from build123d import *

# Parameters (mm, degrees)
SKETCH1_R          = 8
EXTRUDE1_DEPTH     = 1102
SKETCH3_R          = 8
SKETCH3_R_2        = 6
CUT_EXTRUDE1_DEPTH = 54
SKETCH4_R          = 8
SKETCH4_R_2        = 6
CUT_EXTRUDE2_DEPTH = 20
SKETCH5_R          = 6
EXTRUDE2_DEPTH     = 4.4
SKETCH6_R          = 8
SKETCH6_R_2        = 6
EXTRUDE3_DEPTH     = 3
SKETCH7_R          = 8
SKETCH7_R_2        = 6
EXTRUDE4_DEPTH     = 3


with BuildPart() as part:
    # Sketch1 → Extrude1 (new body)
    with BuildSketch(Plane.XY):
        Circle(SKETCH1_R)
    extrude(amount=EXTRUDE1_DEPTH)

    # Sketch3 → Cut-Extrude1 (cut)
    with BuildSketch(Plane.XY.offset(1102)):
        Circle(SKETCH3_R)
        Circle(SKETCH3_R_2, mode=Mode.SUBTRACT)
    extrude(amount=-CUT_EXTRUDE1_DEPTH, mode=Mode.SUBTRACT)

    # Sketch4 → Cut-Extrude2 (cut)
    with BuildSketch(Plane(origin=(0, 0, 0), x_dir=(-1, 0, 0), z_dir=(0, 0, -1))):
        Circle(SKETCH4_R)
        Circle(SKETCH4_R_2, mode=Mode.SUBTRACT)
    extrude(amount=-CUT_EXTRUDE2_DEPTH, mode=Mode.SUBTRACT)

    # Sketch5 → Extrude2 (add)
    with BuildSketch(Plane.XY.offset(1102)):
        Circle(SKETCH5_R)
    extrude(amount=EXTRUDE2_DEPTH)

    # Sketch6 → Extrude3 (add)
    with BuildSketch(Plane.XY.offset(1048)):
        Circle(SKETCH6_R)
        Circle(SKETCH6_R_2, mode=Mode.SUBTRACT)
    extrude(amount=EXTRUDE3_DEPTH)

    # Sketch7 → Extrude4 (add)
    with BuildSketch(Plane(origin=(0, 0, 20), x_dir=(-1, 0, 0), z_dir=(0, 0, -1))):
        Circle(SKETCH7_R)
        Circle(SKETCH7_R_2, mode=Mode.SUBTRACT)
    extrude(amount=EXTRUDE4_DEPTH)


solid = part.part
Part model, mm, in its own coordinate system. Coordinates: 2 decimals unless noted, no trailing zeros. Loops run counter-clockwise (first coordinate to the right, second up) from the corner with the lowest first, then second, coordinate; pieces in that order, holes last. Notation, with made-up numbers: (26, 81) -> (75, 81) arc R17 cw to (75, 108) -> close; hole circle Ø6 at (10, 58). An arc over 180 degrees is marked (long way). Use a Markdown table: item, result. Add a question column.
Item 1: Flat gauge pins, fed straight in: P1, Ø5, axis at x = 5, z = 912, coming from the -Y side; P2, Ø2, axis at x = 6, y = 2.5, coming from the +Z side; P3, Ø2, axis at y = -2.5, z = 494.5, coming from the -X side; P4, Ø5, axis at x = 5.5, z = 152, coming from the -Y side. Where does each tip first touch, or does it go through?
Item 2: Band-saw the part on A-A on y = 0. Write the cut outline in (x, z).
Item 3: Probe probe 1 along Y at (x, z) = (1, 474); probe 2 along Y at (x, z) = (-0.75, 523.5). List the from-to ranges inside material, lowest first.
Item 4: Band-saw the part on C-C on z = 879. Write the cut outline in (x, y), plus the area to 3 significant figures.
Geometry says:
| question | item | result |
|---|---|---|
| 1 | P1 | y = -7.6 |
| 1 | P2 | z = 1106.4 |
| 1 | P3 | x = -7.86 |
| 1 | P4 | y = -7.42 |
| 2 | outline | (-8, 17) -> (-6, 17) -> (-6, 0) -> (6, 0) -> (6, 17) -> (8, 17) -> (8, 1051) -> (6, 1051) -> (6, 1106.4) -> (-6, 1106.4) -> (-6, 1051) -> (-8, 1051) -> close |
| 3 | probe 1 | -7.94 to 7.94 |
| 3 | probe 2 | -7.96 to 7.96 |
| 4 | outline | circle Ø16 at (0, 0) |
| 4 | area | 201 mm² |
